Part print with two shaded views. Sizes in mm from the minimum x, y, z corner. A direction names the side the tool comes from. Give positions to 0.01 mm unless a question says otherwise; leave off trailing zeros. Write each loop counter-clockwise with the first axis right and the second up, starting at its lowest first coordinate (ties: lowest second). Pieces come first, ordered by that corner, then holes.
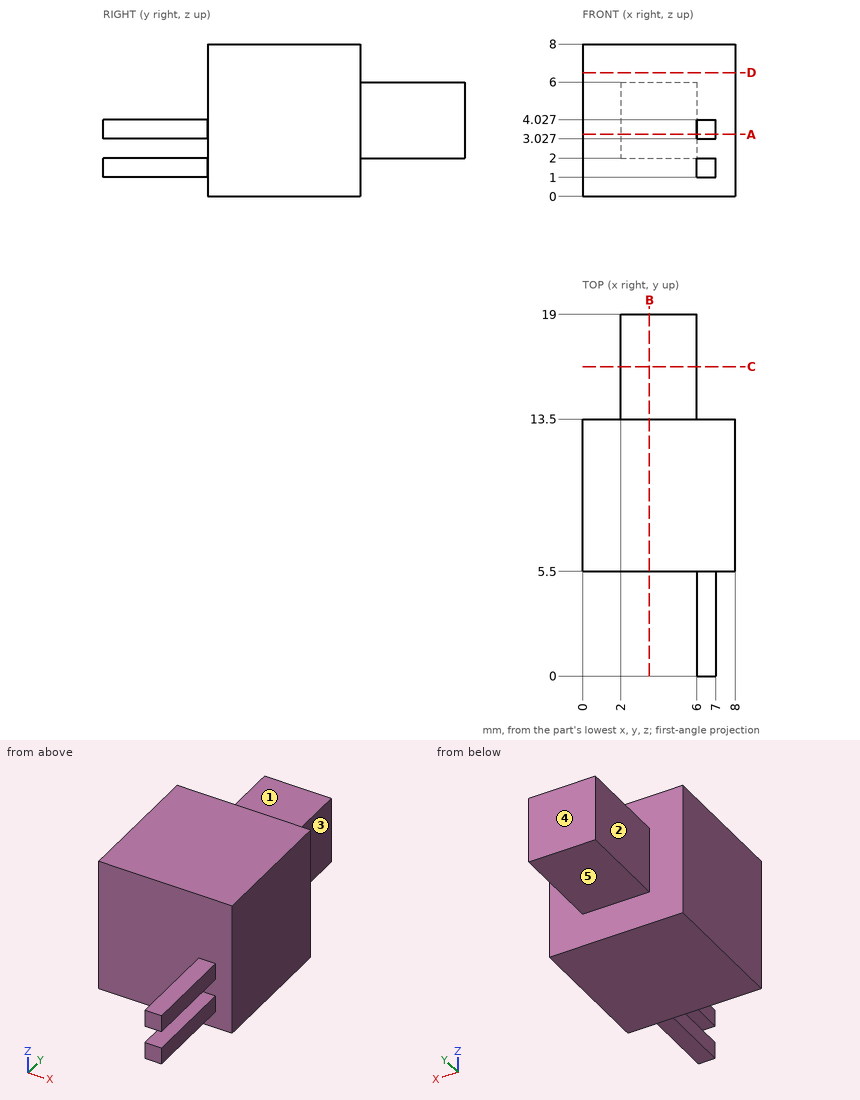
1) Pin check, flat tips, straight feed: pin 1 Ø0.5 at (x, y) = (6.5, 3) entering from -Z; pin 2 Ø0.5 at (y, z) = (1.5, 1.5) entering from -X; pin 3 Ø0.5 at (y, z) = (3, 1.5) entering from +X. Stop position of each tip, or through.
Answers follow:
pin 1: stops at z = 1
pin 2: stops at x = 6
pin 3: stops at x = 7
2) Saw through at D-D, the plane z = 6.5. Write the cut outline in (x, y).
Answers follow:
outline: (0, 5.5) - (8, 5.5) - (8, 13.5) - (0, 13.5) - close
3) 3-axis set-ups, long thin cutter, end or side, ignore diameter. For the marked faces 1, 2, 3, 4 and 5: which of +Z, -Z, +X, -X, +Y, -Y reach the whole face in a straight line?
Answers follow:
face 1: +Z, +X, -X, +Y
face 2: +Z, -Z, -X, +Y
face 3: +Z, -Z, +X, +Y
face 4: +Z, -Z, +X, -X, +Y
face 5: -Z, +X, -X, +Y
4) Saw through at B-B, the plane x = 3.5. Write the cut outline in (y, z).
Answers follow:
outline: (5.5, 0) - (13.5, 0) - (13.5, 2) - (19, 2) - (19, 6) - (13.5, 6) - (13.5, 8) - (5.5, 8) - close
5) Wall check: L1, parallel to Y at x = 5, z = 7.5; L2, parallel to Y at x = 2.5, z = 3.5; L3, parallel to X at y = 17.75, z = 2.5. Give the ranges that are in metal, low to high.
Answers follow:
L1: y = 5.5 to 13.5
L2: y = 5.5 to 19
L3: x = 2 to 6
6) Saw through at C-C, the plane y = 16.25. Write the cut outline in (x, z), then the cut area to 3 significant figures.
Answers follow:
outline: (2, 2) - (6, 2) - (6, 6) - (2, 6) - close
area: 16.0 mm2
7) Saw through at A-A, the plane z = 3.25. Write the cut outline in (x, y), then the cut area to 3 significant figures.
Answers follow:
outline: (0, 5.5) - (6, 5.5) - (6, 0) - (7, 0) - (7, 5.5) - (8, 5.5) - (8, 13.5) - (6, 13.5) - (6, 19) - (2, 19) - (2, 13.5) - (0, 13.5) - close
area: 91.5 mm2
